Input: part model. Units: mm. Frame: model coordinates. A direction names the side the tool comes from. Round coordinates to 2 decimals unless told otherwise and drop trailing zeros. Loops run counter-clockwise (first coordinate to the right, second up) from the corner with the lowest first, then second, coordinate; pieces in that order, holes last.
1) Access query for faces 1 (the face through (52, 37, 35.25)), 2 (the face through (63, 44.75, -10)), 3 (the face through (53, 57, -10)). Directions: +Z, -Z, +X, -X, +Y, -Y. A direction counts if a zero-diameter tool reaches every point of the face in a straight line with its end or side. Return the directions, or none.
2) Draft query along Y for faces 4 (the face through (63, 29.25, -10)), 5 (the face through (44, 8, -32)), 6 (the face through (54.6, 14.4, -25.9)). Return one class per face: pulls with the +Y half, pulls with the -Y half, needs draft (parallel to the pull), parting line crosses it, or undercut.
3) Section B-B, the plane y = 62.5. Return loops of the section in (x, z).
4) Section D-D, the plane x = 0. Return loops of the section in (y, z), and give its area (3 significant figures).
5) First-contact query: pin 1 (2 mm diameter, centred on x = -63, y = 48.5, fed in from -Z); pin 2 (2 mm diameter, centred on x = -32, z = 12, fed in from +Y); pin 3 (4 mm diameter, centred on y = 48, z = 32, fed in from +X); pin 4 (8 mm diameter, centred on x = 51.5, z = -32.5, fed in from +Y). Flat tips, straight axial feed; report the tip coordinate or a pass-through.
6) Ray query, line 1 along Y through (x, z) = (-63, 32); line 2 along Z through (x, y) = (-14, 53.5); line 3 along X through (y, z) = (49, -17.5). Return the intervals inside material, ascending.
7) Section A-A, the plane z = 0. Return loops of the section in (x, y).
8) Section C-C, the plane x = -24. Return loops of the section in (y, z).
from build123d import *

# Parameters (mm, degrees)
SKETCH1_W               = 80
SKETCH1_H               = 80
SKETCH1_R               = 18.4
BOSS_EXTRUDE1_DEPTH     = 2
SKETCH2_W               = 4
SKETCH2_H               = 18.5
BOSS_EXTRUDE2_DEPTH     = 15.25
SKETCH3_R               = 2.2
CUT_EXTRUDE1_DEPTH      = 94.976393312
MIRROR2_COPY_1_SKETCH_W = 4
MIRROR2_COPY_1_SKETCH_H = 18.5
MIRROR2_COPY_1_DEPTH    = 15.25
MIRROR2_COPY_2_SKETCH_R = 2.2
MIRROR2_COPY_2_DEPTH    = 94.976393312
SKETCH4_R               = 2.2
CUT_EXTRUDE2_DEPTH      = 62.388618652
SKETCH5_W               = 4
SKETCH5_H               = 15.25
CUT_EXTRUDE3_DEPTH      = 93.258129723
SKETCH6_W               = 80
SKETCH6_H               = 80
SKETCH6_W_2             = 76
SKETCH6_H_2             = 76
BOSS_EXTRUDE3_DEPTH     = 75
SKETCH7_W               = 25
SKETCH7_H               = 77
BOSS_EXTRUDE4_DEPTH     = 80
CUT_EXTRUDE5_DEPTH      = 21
SKETCH11_W              = 25
SKETCH11_H              = 40
CUT_EXTRUDE6_DEPTH      = 50
BOSS_EXTRUDE5_DEPTH     = 25
SKETCH14_W              = 46.5
SKETCH14_H              = 28.5
SKETCH14_R              = 10.25
CUT_EXTRUDE9_DEPTH      = 34
SKETCH15_W              = 6.5
SKETCH15_H              = 6.5
SKETCH15_R              = 2.45
BOSS_EXTRUDE6_DEPTH     = 4


with BuildPart() as part:
    # Sketch1 → Boss-Extrude1 (new body)
    with BuildSketch(Plane(origin=(0, 0, 0), x_dir=(1, 0, 0), z_dir=(0, 1, 0))):
        Rectangle(SKETCH1_W, SKETCH1_H)
        with Locations(Location((0, 0, 0), (0, 0, 270))):
            Circle(SKETCH1_R, mode=Mode.SUBTRACT)
    extrude(amount=BOSS_EXTRUDE1_DEPTH)

    # Sketch2 → Boss-Extrude2 (add)
    with BuildSketch(Plane(origin=(0, 2, 0), x_dir=(1, 0, 0), z_dir=(0, 1, 0))):
        with Locations((42, -30.75)):
            Rectangle(SKETCH2_W, SKETCH2_H)
    boss_extrude2 = extrude(amount=-BOSS_EXTRUDE2_DEPTH)

    # Sketch3 → Cut-Extrude1 (cut, through all)
    with BuildSketch(Plane(origin=(44, 0, 0), x_dir=(0, 0, -1), z_dir=(1, 0, 0))):
        with Locations((-30.75, -8.125)):
            Circle(SKETCH3_R)
    cut_extrude1 = extrude(amount=-CUT_EXTRUDE1_DEPTH, mode=Mode.SUBTRACT)

    # Mirror1: Boss-Extrude2, Cut-Extrude1 across plane
    add(boss_extrude2.mirror(Plane(origin=(0, 0, 0), x_dir=(0, 0, 1), z_dir=(1, 0, 0))))
    add(cut_extrude1.mirror(Plane(origin=(0, 0, 0), x_dir=(0, 0, 1), z_dir=(1, 0, 0))), mode=Mode.SUBTRACT)

    # Mirror2: Boss-Extrude2, Cut-Extrude1 across plane
    add(boss_extrude2.mirror(Plane(origin=(0, 0, 0), x_dir=(1, 0, 0), z_dir=(0, 0, -1))))
    add(cut_extrude1.mirror(Plane(origin=(0, 0, 0), x_dir=(1, 0, 0), z_dir=(0, 0, -1))), mode=Mode.SUBTRACT)

    # Mirror2 copy 1 sketch → Mirror2 copy 1 (add)
    with BuildSketch(Plane(origin=(0, 2, 0), x_dir=(-1, 0, 0), z_dir=(0, 1, 0))):
        with Locations((42, -30.75)):
            Rectangle(MIRROR2_COPY_1_SKETCH_W, MIRROR2_COPY_1_SKETCH_H)
    extrude(amount=-MIRROR2_COPY_1_DEPTH)

    # Mirror2 copy 2 sketch → Mirror2 copy 2 (cut, through all)
    with BuildSketch(Plane.ZY.offset(44)):
        with Locations((-30.75, -8.125)):
            Circle(MIRROR2_COPY_2_SKETCH_R)
    extrude(amount=-MIRROR2_COPY_2_DEPTH, mode=Mode.SUBTRACT)

    # Sketch4 → Cut-Extrude2 (cut, through all)
    with BuildSketch(Plane(origin=(0, 2, 0), x_dir=(1, 0, 0), z_dir=(0, 1, 0))):
        with Locations(Location((-24, 24, 0), (0, 0, 270))):
            Circle(SKETCH4_R)
        with Locations(Location((24, 24, 0), (0, 0, 270))):
            Circle(SKETCH4_R)
    cut_extrude2 = extrude(amount=-CUT_EXTRUDE2_DEPTH, mode=Mode.SUBTRACT)

    # Mirror3: Cut-Extrude2 across plane
    add(cut_extrude2.mirror(Plane(origin=(0, 0, 0), x_dir=(1, 0, 0), z_dir=(0, 0, -1))), mode=Mode.SUBTRACT)

    # Sketch5 → Cut-Extrude3 (cut, through all)
    with BuildSketch(Plane.XY.offset(40)):
        with Locations((-42, -5.625)):
            Rectangle(SKETCH5_W, SKETCH5_H)
        with Locations((42, -5.625)):
            Rectangle(SKETCH5_W, SKETCH5_H)
    extrude(amount=-CUT_EXTRUDE3_DEPTH, mode=Mode.SUBTRACT)

    # Sketch6 → Boss-Extrude3 (add)
    with BuildSketch(Plane(origin=(0, 2, 0), x_dir=(1, 0, 0), z_dir=(0, 1, 0))):
        Rectangle(SKETCH6_W, SKETCH6_H)
        Rectangle(SKETCH6_W_2, SKETCH6_H_2, mode=Mode.SUBTRACT)
    extrude(amount=BOSS_EXTRUDE3_DEPTH)

    # Sketch7 → Boss-Extrude4 (add)
    with BuildSketch(Plane.XY.offset(40)):
        with Locations((-52.5, 38.5)):
            Rectangle(SKETCH7_W, SKETCH7_H)
        with Locations((52.5, 38.5)):
            Rectangle(SKETCH7_W, SKETCH7_H)
    extrude(amount=-BOSS_EXTRUDE4_DEPTH)

    # Sketch9 → Cut-Extrude5 (cut)
    with BuildSketch(Plane(origin=(65, 0, 0), x_dir=(0, 0, -1), z_dir=(1, 0, 0))):
        Polygon((40, 0), (40, 28.5), (11.5, 0), align=None)
    cut_extrude5 = extrude(amount=-CUT_EXTRUDE5_DEPTH, mode=Mode.SUBTRACT)

    # Mirror4: Cut-Extrude5 across plane
    add(cut_extrude5.mirror(Plane(origin=(0, 0, 0), x_dir=(0, 0, 1), z_dir=(1, 0, 0))), mode=Mode.SUBTRACT)

    # Sketch11 → Cut-Extrude6 (cut)
    with BuildSketch(Plane(origin=(0, 0, -40), x_dir=(-1, 0, 0), z_dir=(0, 0, -1))):
        with Locations((-52.5, 57)):
            Rectangle(SKETCH11_W, SKETCH11_H)
        with Locations((52.5, 57)):
            Rectangle(SKETCH11_W, SKETCH11_H)
    extrude(amount=-CUT_EXTRUDE6_DEPTH, mode=Mode.SUBTRACT)

    # Sketch12 → Boss-Extrude5 (add)
    with BuildSketch(Plane(origin=(65, 0, 0), x_dir=(0, 0, -1), z_dir=(1, 0, 0))):
        Polygon((30, 37), (-10, 77), (-10, 37), align=None)
    boss_extrude5 = extrude(amount=-BOSS_EXTRUDE5_DEPTH)

    # Mirror5: Boss-Extrude5 across plane
    add(boss_extrude5.mirror(Plane(origin=(0, 0, 0), x_dir=(0, 0, 1), z_dir=(1, 0, 0))))

    # Sketch14 → Cut-Extrude9 (cut)
    # profile 1 of 2: a face of its own
    with BuildSketch(Plane(origin=(65, 0, 0), x_dir=(0, 0, -1), z_dir=(1, 0, 0))):
        with Locations((-12, 37)):
            Rectangle(SKETCH14_W, SKETCH14_H)
        with Locations((0, 37)):
            Circle(SKETCH14_R, mode=Mode.SUBTRACT)
    # profile 2 of 2: a face of its own
    with BuildSketch(Plane(origin=(65, 0, 0), x_dir=(0, 0, -1), z_dir=(1, 0, 0))):
        with Locations((0, 37)):
            Circle(SKETCH14_R)
    cut_extrude9 = extrude(amount=-CUT_EXTRUDE9_DEPTH, mode=Mode.SUBTRACT)

    # Mirror6: Cut-Extrude9 across plane
    add(cut_extrude9.mirror(Plane(origin=(0, 0, 0), x_dir=(0, 0, 1), z_dir=(1, 0, 0))), mode=Mode.SUBTRACT)

    # Sketch15 → Boss-Extrude6 (add)
    # profile 1 of 4: a face of its own
    with BuildSketch(Plane(origin=(65, 0, 0), x_dir=(0, 0, -1), z_dir=(1, 0, 0))):
        with Locations((-32, 48)):
            Rectangle(SKETCH15_W, SKETCH15_H)
        with Locations((-32, 48)):
            Circle(SKETCH15_R, mode=Mode.SUBTRACT)
    # profile 2 of 4: a face of its own
    with BuildSketch(Plane(origin=(65, 0, 0), x_dir=(0, 0, -1), z_dir=(1, 0, 0))):
        with Locations((-32, 26)):
            Rectangle(SKETCH15_W, SKETCH15_H)
        with Locations((-32, 26)):
            Circle(SKETCH15_R, mode=Mode.SUBTRACT)
    # profile 3 of 4: a face of its own
    with BuildSketch(Plane(origin=(65, 0, 0), x_dir=(0, 0, -1), z_dir=(1, 0, 0))):
        with BuildLine():
            ThreePointArc((7.806247498, 29.25), (6.371323573, 28.033047567), (4.75, 27.078432584))
            Line((4.75, 27.078432584), (4.75, 22.75))
            Line((4.75, 22.75), (11.25, 22.75))
            Line((11.25, 22.75), (11.25, 29.25))
            Line((11.25, 29.25), (7.806247498, 29.25))
        make_face()
        with Locations((8, 26)):
            Circle(SKETCH15_R, mode=Mode.SUBTRACT)
    # profile 4 of 4: a face of its own
    with BuildSketch(Plane(origin=(65, 0, 0), x_dir=(0, 0, -1), z_dir=(1, 0, 0))):
        with BuildLine():
            Line((11.25, 51.25), (4.75, 51.25))
            Line((4.75, 51.25), (4.75, 46.921567416))
            ThreePointArc((4.75, 46.921567416), (6.371323573, 45.966952433), (7.806247498, 44.75))
            Line((7.806247498, 44.75), (11.25, 44.75))
            Line((11.25, 44.75), (11.25, 51.25))
        make_face()
        with Locations((8, 48)):
            Circle(SKETCH15_R, mode=Mode.SUBTRACT)
    boss_extrude6 = extrude(amount=-BOSS_EXTRUDE6_DEPTH)

    # Mirror7: Boss-Extrude6 across plane
    add(boss_extrude6.mirror(Plane(origin=(0, 0, 0), x_dir=(0, 0, 1), z_dir=(1, 0, 0))))


solid = part.part
Final values:
1. face 1: none
1. face 2: +X, -X
1. face 3: -Z, +X, +Y
2. face 4: undercut
2. face 5: needs draft
2. face 6: pulls with the -Y half
3. outline: (-65, -4.5) - (-40, -4.5) - (-40, -40) - (40, -40) - (40, -4.5) - (65, -4.5) - (65, 40) - (-65, 40) - close; hole (-38, -38) - (38, -38) - (38, 38) - (-38, 38) - close
4. outline: (0, -40) - (77, -40) - (77, -38) - (2, -38) - (2, -18.4) - (0, -18.4) - close; (0, 18.4) - (2, 18.4) - (2, 38) - (77, 38) - (77, 40) - (0, 40) - close
4. area: 386 mm2
5. pin 1: stops at z = -19.5
5. pin 2: stops at y = 2
5. pin 3: passes through
5. pin 4: stops at y = 38.5
6. line 1: y = 0 to 23.55, 28.45 to 29.25, 44.75 to 45.55, 50.45 to 77
6. line 2: z = -40 to -38, 38 to 40
6. line 3: x = -65 to -38, 38 to 65
7. outline: (-65, 0) - (-18.4, 0) - (-18.4, 2) - (-38, 2) - (-38, 22.75) - (-65, 22.75) - close; (-65, 51.25) - (-38, 51.25) - (-38, 77) - (-40, 77) - (-40, 67) - (-65, 67) - close; (18.4, 0) - (65, 0) - (65, 22.75) - (38, 22.75) - (38, 2) - (18.4, 2) - close; (38, 51.25) - (65, 51.25) - (65, 67) - (40, 67) - (40, 77) - (38, 77) - close
8. outline: (0, -40) - (77, -40) - (77, -38) - (2, -38) - (2, -26.2) - (0, -26.2) - close; (0, -21.8) - (2, -21.8) - (2, 21.8) - (0, 21.8) - close; (0, 26.2) - (2, 26.2) - (2, 38) - (77, 38) - (77, 40) - (0, 40) - close
